```python
from build123d import *

# Parameters (mm, degrees)
BOSS_EXTRUDE1_DEPTH = 2
FILLET1_R           = 0.8
FILLET2_R           = 2
CUT_EXTRUDE1_DEPTH  = 15.121515427
CHAMFER1_SIZE       = 1.2


with BuildPart() as part:
    # Sketch1 → Boss-Extrude1 (new body)
    with BuildSketch(Plane.XY):
        Polygon((5.802857873, 2.85130668), (0.3, 7.45130668), (0.3, 9.45130668), (8.195404775, 2.85130668), (8.195404775, -0.14869332), (0.3, -6.74869332), (0.3, -4.74869332), (5.802857873, -0.14869332), (-2.7, -0.14869332), (-2.7, -1.34869332), (-4.7, -1.34869332), (-4.7, -0.14869332), (-10.3, -0.14869332), (-10.3, 2.85130668), (-3.3, 9.45130668), (-0.3, 9.45130668), (-0.3, 2.85130668), align=None)
    extrude(amount=BOSS_EXTRUDE1_DEPTH)

    # Fillet1
    fillet1_edges = [part.edges().sort_by_distance(p)[0] for p in [
        (0.3, 9.45130668, 1),
        (0.3, -6.74869332, 1),
    ]]
    fillet(fillet1_edges, radius=FILLET1_R)

    # Fillet2
    fillet2_edges = [part.edges().sort_by_distance(p)[0] for p in [
        (-10.3, 2.85130668, 1),
        (-3.3, 9.45130668, 1),
        (8.195404775, 2.85130668, 1),
        (8.195404775, -0.14869332, 1),
    ]]
    fillet(fillet2_edges, radius=FILLET2_R)

    # Sketch2 → Cut-Extrude1 (cut, through all)
    with BuildSketch(Plane.XY.offset(2)):
        Polygon((-1.383139325, 7.45130668), (-1.383139325, -0.14869332), (-1.863442011, -0.14869332), (-1.863442011, 0.979922786), (-8.3, 0.979922786), (-8.3, 1.988217887), (-2.505814916, 7.45130668), align=None)
    extrude(amount=-CUT_EXTRUDE1_DEPTH, mode=Mode.SUBTRACT)

    # Chamfer1
    chamfer1_edges = [part.edges().sort_by_distance(p)[0] for p in [
        (-4.7, -1.34869332, 1),
    ]]
    chamfer(chamfer1_edges, length=CHAMFER1_SIZE - 0.0001)  # a hair under: the kernel refuses the full size


solid = part.part
```
Geometry: final body of the model. Coordinates: model frame, mm. A direction names the side the tool comes from. Coordinates: 2 decimals unless noted, no trailing zeros. Order: outer loops, then holes, each group sorted by start corner. A loop starts at its lowest first (then second) coordinate and runs counter-clockwise, first axis right, second up. Notation, with made-up numbers: (-24.75, -1.5) - (11.25, -1.5) arc R30 ccw to (11.25, 31.5) - close; hole circle Ø5 at (-2.5, 2.5). An arc over 180 degrees is marked (long way). Return JSON: item names as keys, results as strings. Group by question number.
1. Cut plane A-A (y = -0.5). Output: boundary loops of the cut face in (x, z), plus the area to 3 significant figures.
2. Pull-direction query (Y, two-part tool) for faces 5 (the face through (3.09, 5.12, 0.99)), 6 (the face through (0.75, 8.46, 1.01)), 7 (the face through (-2.7, -1, 1)); classes: pulls with the +Y half, pulls with the -Y half, needs draft (parallel to the pull), parting line crosses it, or undercut.
3. Set-up query: faces 1 (the face through (-5.443, 4.682, 1.014)), 2 (the face through (-0.3, 6, 1)), 3 (the face through (-2.3, -0.149, 1)), 4 (the face through (-3, -1.349, 1)). Return all of +Z, -Z, +X, -X, +Y, -Y with unobstructed straight access to the full face (end or side cutting, diameter ignored); none if empty.
4. Material intervals for line 1 along X through (y, z) = (1.5, 0.25); line 2 along X through (y, z) = (4, 0.8); line 3 along X through (y, z) = (0.75, 0.6), sorted ascending. Write a range as [from, to].
5. Cut plane D-D (y = 7). Output: boundary loops of the cut face in (x, z).
6. Pin query (flat end, axial travel): pin 1 (1 mm diameter, centred on y = 6.5, z = 1.5, fed in from +X); pin 2 (0.9 mm diameter, centred on x = -2, z = 1, fed in from -Y); pin 3 (0.6 mm diameter, centred on x = 4, z = 1.5, fed in from +Y). Return the tip coordinate at first contact, or that it passes through.
7. Cut plane C-C (x = 1). Output: boundary loops of the cut face in (y, z).
Resolved:
{
 "1": {"outline": "(-4.35, 0) - (-2.7, 0) - (-2.7, 2) - (-4.35, 2) - close; (5.38, 0) - (7.73, 0) - (7.73, 2) - (5.38, 2) - close", "area": "7.99 mm²"},
 "2": {"face 5": "undercut", "face 6": "pulls with the +Y half", "face 7": "needs draft"},
 "3": {"face 1": "+Z, -Z", "face 2": "+Z, -Z, +Y", "face 3": "+Z, -Z, -Y", "face 4": "+Z, -Z, -X, -Y"},
 "4": {"line 1": "x = [-10.3, -8.3], [-1.38, 8.2]", "line 2": "x = [-9.08, -6.17], [-1.38, -0.3], [4.43, 6.82]", "line 3": "x = [-10.3, -1.86], [-1.38, 8.2]"},
 "5": {"outline": "(-5.9, 0) - (-2.98, 0) - (-2.98, 2) - (-5.9, 2) - close; (-1.38, 0) - (-0.3, 0) - (-0.3, 2) - (-1.38, 2) - close; (0.84, 0) - (3.23, 0) - (3.23, 2) - (0.84, 2) - close"},
 "6": {"pin 1": "stops at x = 4.43", "pin 2": "stops at y = -0.15", "pin 3": "stops at y = 6.61"},
 "7": {"outline": "(-5.83, 0) - (-4.16, 0) - (-4.16, 2) - (-5.83, 2) - close; (-0.15, 0) - (2.85, 0) - (2.85, 2) - (-0.15, 2) - close; (6.87, 0) - (8.53, 0) - (8.53, 2) - (6.87, 2) - close"}
}
